Check sheet for the modelled part. Datum: model origin and axes. Units: mm. Face numbers are marked on the shaded views. A direction names the side the tool comes from. Give positions to 0.01 mm unless a question says otherwise; leave off trailing zeros. Loops run counter-clockwise (first coordinate to the right, second up) from the corner with the lowest first, then second, coordinate; pieces in that order, holes last. Notation, with made-up numbers: M 5,26 L 43,26 A12 ccw 43,37 Z; hole C 10.25,29.25 d8. An arc over 180 degrees is marked long. Use one line per item in the form item = value.
from build123d import *

# Parameters (mm, degrees)
SKETCH4_R           = 3.96875
SKETCH4_R_2         = 5.2959
SKETCH4_R_3         = 1.5
SKETCH4_R_4         = 3.175
BOSS_EXTRUDE2_DEPTH = 10.16


with BuildPart() as part:
    # Sketch4 → Boss-Extrude2 (new body)
    with BuildSketch(Plane(origin=(0, 0, 0), x_dir=(1, 0, 0), z_dir=(0, 1, 0))):
        with BuildLine():
            Line((54.2925, 31.75), (-12.3825, 31.75))
            Line((-12.3825, 31.75), (-8.838261623, -0.957722033))
            ThreePointArc((-8.838261623, -0.957722033), (-4.569283935, -7.625860235), (3.324048375, -8.245168428))
            Line((3.324048375, -8.245168428), (19.191308787, -1.848265606))
            ThreePointArc((19.191308787, -1.848265606), (19.706480828, -1.70147711), (20.240980706, -1.665995068))
            Line((20.240980706, -1.665995068), (31.935252388, -2.1264974))
            ThreePointArc((31.935252388, -2.1264974), (32.505817446, -2.214628745), (33.041741732, -2.429330346))
            Line((33.041741732, -2.429330346), (38.89391711, -5.588))
            ThreePointArc((38.89391711, -5.588), (44.459162112, -5.815863868), (48.063098072, -1.569039233))
            Line((48.063098072, -1.569039233), (54.2925, 22.86))
            Line((54.2925, 22.86), (54.2925, 31.75))
        make_face()
        with Locations(Location((0, 0, 0), (0, 0, 270))):
            Circle(SKETCH4_R, mode=Mode.SUBTRACT)
        with Locations(Location((46.355, 22.86, 0), (0, 0, 270))):
            Circle(SKETCH4_R, mode=Mode.SUBTRACT)
        with Locations(Location((-4.445, 22.86, 0), (0, 0, 270))):
            Circle(SKETCH4_R, mode=Mode.SUBTRACT)
        with Locations(Location((16.764, 8.636, 0), (0, 0, 270))):
            Circle(SKETCH4_R_2, mode=Mode.SUBTRACT)
        with Locations(Location((27.264, 8.636, 0), (0, 0, 270))):
            Circle(SKETCH4_R_3, mode=Mode.SUBTRACT)
        with Locations(Location((6.264, 8.636, 0), (0, 0, 270))):
            Circle(SKETCH4_R_3, mode=Mode.SUBTRACT)
        with Locations(Location((41.91, 0, 0), (0, 0, 270))):
            Circle(SKETCH4_R_4, mode=Mode.SUBTRACT)
        with BuildLine():
            Line((40.788789755, 27.94), (8.256445186, 27.94))
            ThreePointArc((8.256445186, 27.94), (8.029131858, 27.799334245), (8.053591766, 27.533138984))
            Line((8.053591766, 27.533138984), (12.594862372, 21.506669344))
            ThreePointArc((12.594862372, 21.506669344), (13.490054122, 20.762146224), (14.623396567, 20.495279502))
            Line((14.623396567, 20.495279502), (19.573752381, 20.495279502))
            ThreePointArc((19.573752381, 20.495279502), (20.231152756, 20.408731101), (20.843752381, 20.154984028))
            Line((20.843752381, 20.154984028), (24.06434333, 18.295574977))
            ThreePointArc((24.06434333, 18.295574977), (24.676942955, 18.041827904), (25.33434333, 17.955279502))
            Line((25.33434333, 17.955279502), (30.365177054, 17.955279502))
            ThreePointArc((30.365177054, 17.955279502), (31.337192972, 18.14862549), (32.161228278, 18.699228278))
            Line((32.161228278, 18.699228278), (40.968394878, 27.506394878))
            ThreePointArc((40.968394878, 27.506394878), (41.023455156, 27.783201592), (40.788789755, 27.94))
        make_face(mode=Mode.SUBTRACT)
    extrude(amount=BOSS_EXTRUDE2_DEPTH)


solid = part.part
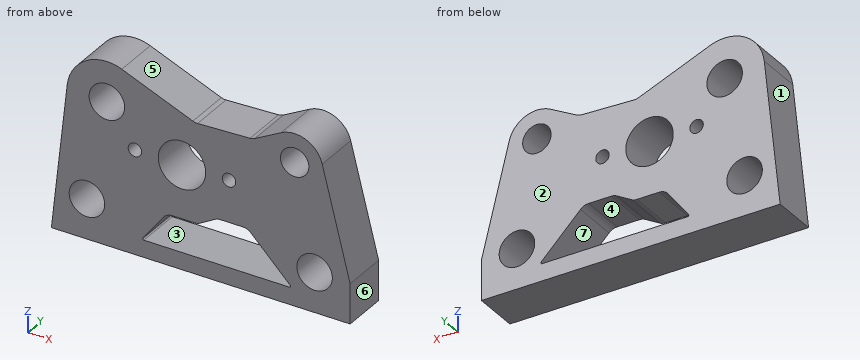
1) Section check A-A (z = -24). Record the cut outline in (x, y).
Evaluation:
outline = M -11.54,0 L -8.25,0 L -8.25,10.16 L -11.54,10.16 Z; M -0.64,0 L 10.72,0 L 10.72,10.16 L -0.64,10.16 Z; M 37.46,0 L 42.55,0 L 42.55,10.16 L 37.46,10.16 Z; M 50.16,0 L 54.29,0 L 54.29,10.16 L 50.16,10.16 Z
2) Section check C-C (z = -5.5). Record the cut outline in (x, y).
Evaluation:
outline = M -9.54,0 L 12.5,0 L 12.5,10.16 L -9.54,10.16 Z; M 21.03,0 L 49.87,0 L 49.87,10.16 L 21.03,10.16 Z
3) Set-up check for the marked faces 5, 6 and 7: record each of +Z, -Z, +X, -X, +Y, -Y from which the full face is reachable in a straight line by a thin tool's end or side.
Evaluation:
face_5 = +Z, +Y, -Y
face_6 = +Z, -Z, +X, +Y, -Y
face_7 = +Y, -Y
4) Section check D-D (y = 9). State how many separate pieces and enclosed holes the cut face has, then the cut area to 3 significant figures.
Evaluation:
separate_pieces = 1
enclosed_holes = 8
area = 1,760 mm^2
5) Release check for a two-part mould opening along X. For the marked faces 1, 2, 3 and 4 record: pulls with the +X half, pulls with the -X half, needs draft (parallel to the pull), parting line crosses it, or undercut.
Evaluation:
face_1 = pulls with the -X half
face_2 = needs draft
face_3 = undercut
face_4 = undercut
6) Section check B-B (x = -7.5). Record the cut outline in (y, z), then the cut area to 3 significant figures.
Evaluation:
outline = M 0,-31.75 L 10.16,-31.75 L 10.16,-25.39 L 0,-25.39 Z; M 0,-20.33 L 10.16,-20.33 L 10.16,4.77 L 0,4.77 Z
area = 320 mm^2
7) Depth check by flat-ended pin: pin 1 Ø3 at (x, y) = (18.5, 5.5) entering from +Z; pin 2 Ø8 at (x, z) = (17, -25.5) entering from +Y; pin 3 Ø4 at (y, z) = (6.5, -6) entering from -X; pin 4 Ø1 at (y, z) = (6, -15.5) entering from +X. Enter the tip coordinate at first touch or a pass-through.
Evaluation:
pin_1 = 2.73
pin_2 = 10.16
pin_3 = -9.81
pin_4 = 52.54
8) Scan lines: line 1 (Z direction, x = -3, y = 7.5); line 2 (X direction, y = 4.5, z = -22.86); line 3 (Z direction, x = 20, y = 5.5). Record each from-to range of solid material in increasing order.
Evaluation:
line_1 = -31.75 to -26.56, -19.16 to -2.6, 2.6 to 8.37
line_2 = -11.42 to -8.41, -0.48 to 11.58, 36.32 to 42.39, 50.32 to 54.29
line_3 = -31.75 to -27.94, -20.46 to -12.83, -4.44 to 1.67
